Autodesk Fusion 360 part; units mm, degrees
sketch "Sketch1" plane through (0, 0, 0) normal (0, 0, 1) x (1, 0, 0)
  line L0 (-2.5, 5) -> (2.5, 5)
  line L1 (2.5, 5) -> (2.5, -5)
  line L2 (2.5, -5) -> (-2.5, -5)
  line L3 (-2.5, -5) -> (-2.5, 5)
  line L4 (-2.5, 5) -> (2.5, -5) construction
  line L5 (2.5, 5) -> (-2.5, -5) construction
  dimension "d1" = 5
  dimension "d2" = 10
extrude "Extrude1" add sketch "Sketch1" along normal blind 6
ref_plane "WorkPlane1" through (-2.5, 0, 3) normal (-1, 0, 0) x (0, -1, 0)
sketch "Sketch2" plane through (-2.5, 0, 0) normal (-1, 0, 0) x (0, -1, 0)
  line L0 (-2, 0) -> (2, 0)
  line L1 (2, 0) -> (2, 3)
  line L2 (2, 3) -> (-2, 3)
  line L3 (-2, 3) -> (-2, 0)
  dimension "d6" = 4
  dimension "d7" = 3
extrude "Extrude2" cut sketch "Sketch2" against normal blind 6
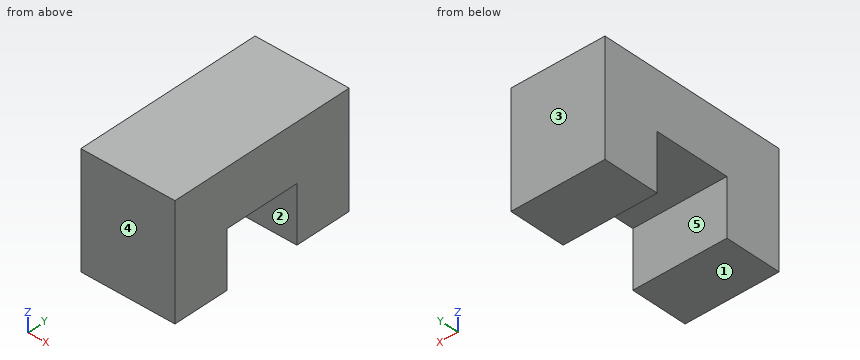
The model under review builds one solid part; all positions refer to its coordinate system, in mm. Face numbers are marked on the shaded views. A direction names the side the tool comes from. Give positions to 0.01 mm unless a question says otherwise; leave off trailing zeros. Write each loop counter-clockwise with the first axis right and the second up, starting at its lowest first coordinate (ties: lowest second). Pieces come first, ordered by that corner, then holes.
1. Add section A-A, the plane z = 1.3. Write out the cut boundary in (x, y), plus the area to 3 significant figures.
2. Wall thickness on L1, parallel to Y at x = 1.3, z = 0.5; L2, parallel to Z at x = -0.7, y = -1: over which ranges is each line inside the solid? List them lowest first.
3. Tool access review of the marked faces 4 and 5: name each direction out of +Z, -Z, +X, -X, +Y, -Y from which nothing blocks a thin tool from reaching the whole face with its end or side.
4. For P1, Ø3, axis at x = 0.5, y = 0, coming from the -Z side, flat-tipped, find the tip position at first contact; note if it passes through.
5. Add section C-C, the plane y = -0.5. Write out the cut boundary in (x, z), plus the area to 3 significant figures.
6. Draft analysis for pull direction Y (two halves, no side actions). For the marked faces 1, 2 and 3, state which applies: +Y half, -Y half, draft (parallel to the pull), parting line (faces both ways), or undercut.
7. Add section B-B, the plane x = 1.9. Write out the cut boundary in (y, z), plus the area to 3 significant figures.
Worked answers:
1. outline: (-2.5, -5) - (2.5, -5) - (2.5, -2) - (-2.5, -2) - close; (-2.5, 2) - (2.5, 2) - (2.5, 5) - (-2.5, 5) - close
1. area: 30.0 mm2
2. L1: y = -5 to -2, 2 to 5
2. L2: z = 3 to 6
3. face 4: +Z, -Z, +X, -X, -Y
3. face 5: -Z, +X, -X
4. P1: stops at z = 3
5. outline: (-2.5, 3) - (2.5, 3) - (2.5, 6) - (-2.5, 6) - close
5. area: 15.0 mm2
6. face 1: draft
6. face 2: undercut
6. face 3: +Y half
7. outline: (-5, 0) - (-2, 0) - (-2, 3) - (2, 3) - (2, 0) - (5, 0) - (5, 6) - (-5, 6) - close
7. area: 48.0 mm2
